Here's how the part is built. I have some questions about the finished solid (model axes, mm). A direction names the side the tool comes from. Coordinates: 2 decimals unless noted, no trailing zeros. Loops run counter-clockwise (first coordinate to the right, second up) from the corner with the lowest first, then second, coordinate; pieces in that order, holes last.
```python
from build123d import *

# Parameters (mm, degrees)
SKETCH_10_W         = 15
SKETCH_10_H         = 8
EXTRUDE_7_DEPTH     = 11
CUT_EXTRUDE_4_DEPTH = 11
SKETCH_12_W         = 15
SKETCH_12_H         = 6
EXTRUDE_8_DEPTH     = 6
SKETCH_14_W         = 15
SKETCH_14_H         = 5
EXTRUDE_9_DEPTH     = 4
EXTRUDE_10_DEPTH    = 15
EXTRUDE_11_DEPTH    = 5
SKETCH_19_R         = 1.1
CUT_EXTRUDE_5_DEPTH = 5
EXTRUDE_START       = 0.5
SKETCH_20_R         = 1.5
SKETCH_20_R_2       = 1.1
EXTRUDE_12_DEPTH    = 0.5
SKETCH_21_R         = 1.5
SKETCH_21_R_2       = 1.1
EXTRUDE_13_DEPTH    = 0.5
FILLET_4_R          = 0.5
CHAMFER_1_SIZE      = 4.493554602
CHAMFER_1_SIZE_2    = 2.7
FILLET_7_R          = 2
SKETCH_22_W         = 15
SKETCH_22_H         = 2
EXTRUDE_14_DEPTH    = 6
FILLET_8_R          = 2
FILLET_9_R          = 2


# Some blends are built 0.0001 mm under size
with BuildPart() as part:
    # 草图10 → 凸台-拉伸7 (new body)
    with BuildSketch(Plane.XY):
        with Locations((0, 24.68211788)):
            Rectangle(SKETCH_10_W, SKETCH_10_H)
    extrude(amount=EXTRUDE_7_DEPTH)

    # 草图11 → 切除-拉伸4 (cut)
    with BuildSketch(Plane(origin=(0, 28.68211788, 0), x_dir=(1, 0, 0), z_dir=(0, 1, 0))):
        with BuildLine():
            Line((-3.45, -5), (-3.45, -7))
            ThreePointArc((-3.45, -7), (-5, -8.55), (-6.55, -7))
            Line((-6.55, -7), (-6.55, -5))
            ThreePointArc((-6.55, -5), (-5, -3.45), (-3.45, -5))
        make_face()
        with BuildLine():
            Line((3.45, -5), (3.45, -7))
            ThreePointArc((3.45, -7), (5, -8.55), (6.55, -7))
            Line((6.55, -7), (6.55, -5))
            ThreePointArc((6.55, -5), (5, -3.45), (3.45, -5))
        make_face()
    extrude(amount=-CUT_EXTRUDE_4_DEPTH, mode=Mode.SUBTRACT)

    # 草图12 → 凸台-拉伸8 (add)
    with BuildSketch(Plane.XY.offset(11)):
        with Locations((0, 25.68211788)):
            Rectangle(SKETCH_12_W, SKETCH_12_H)
    extrude(amount=EXTRUDE_8_DEPTH)

    # 草图14 → 凸台-拉伸9 (add)
    with BuildSketch(Plane.XY.offset(17)):
        with Locations((0, 23.5)):
            Rectangle(SKETCH_14_W, SKETCH_14_H)
    extrude(amount=EXTRUDE_9_DEPTH)

    # 草图17 → 凸台-拉伸10 (add)
    with BuildSketch(Plane.ZY.offset(7.5)):
        Polygon((21, 26), (24.535533906, 29.535533906), (28.071067812, 26), (23.071067812, 21), (21, 21), align=None)
    extrude(amount=-EXTRUDE_10_DEPTH)

    # 草图18 → 凸台-拉伸11 (add)
    with BuildSketch(Plane(origin=(0, -1.035533906, 1.035533906), x_dir=(1, 0, 0), z_dir=(0, -0.7071067811865507, 0.7071067811865445))):
        with BuildLine():
            Line((7.5, 38.234018716), (-7.5, 38.234018716))
            ThreePointArc((-7.5, 38.234018716), (0, 45.734018716), (7.5, 38.234018716))
        make_face()
    extrude(amount=-EXTRUDE_11_DEPTH)

    # 草图19 → 切除-拉伸5 (cut)
    with BuildSketch(Plane(origin=(0, -1.035533906, 1.035533906), x_dir=(1, 0, 0), z_dir=(0, -0.7071067811865507, 0.7071067811865445))):
        with Locations(Location((0, 38.234018716, 0), (0, 0, 270))):
            Circle(SKETCH_19_R)
    extrude(amount=-CUT_EXTRUDE_5_DEPTH, mode=Mode.SUBTRACT)

    # 草图20 → 凸台-拉伸12 (add)
    with BuildSketch(Plane(origin=(0, -1.035533906, 1.035533906), x_dir=(1, 0, 0), z_dir=(0, -0.7071067811865507, 0.7071067811865445)).offset(EXTRUDE_START)):
        with Locations(Location((0, 38.234018716, 0), (0, 0, 270))):
            Circle(SKETCH_20_R)
        with Locations(Location((0, 38.234018716, 0), (0, 0, 270))):
            Circle(SKETCH_20_R_2, mode=Mode.SUBTRACT)
    extrude(amount=-EXTRUDE_12_DEPTH)

    # 草图21 → 凸台-拉伸13 (add)
    with BuildSketch(Plane(origin=(0, 2.5, -2.5), x_dir=(1, 0, 0), z_dir=(0, 0.7071067811865513, -0.7071067811865437))):
        with Locations(Location((0, -38.234018716, 0), (0, 0, 90))):
            Circle(SKETCH_21_R)
        with Locations(Location((0, -38.234018716, 0), (0, 0, 90))):
            Circle(SKETCH_21_R_2, mode=Mode.SUBTRACT)
    extrude(amount=EXTRUDE_13_DEPTH)

    # 圆角4
    fillet_4_edges = [part.edges().sort_by_distance(p)[0] for p in [
        (0, 27.060660172, 29.131727984),
        (0, 30.596194078, 25.596194078),
    ]]
    fillet(fillet_4_edges, radius=FILLET_4_R - 0.0001)  # a hair under: the kernel refuses the full size

    # 倒角1
    # the kernel refuses this chamfer: 4.493554602, 2.7 mm, written as the material it adds along each edge
    with BuildSketch(Plane(origin=(-7.5, 26, 17), x_dir=(0, -0.01991463058083334, 0.9998016840798123), z_dir=(1, 0, 0))) as chamfer_1_piece_1_section:
        Polygon((CHAMFER_1_SIZE * 0.999801684157, -CHAMFER_1_SIZE * 0.0199146305824), (-CHAMFER_1_SIZE_2 * 0.0199146305808, -CHAMFER_1_SIZE_2 * 0.99980168408), (0, 0), align=None)
    chamfer_1_piece_1 = extrude(amount=15, mode=Mode.PRIVATE)
    chamfer_1_piece_1 = split(chamfer_1_piece_1, bisect_by=Plane(origin=(0, 28.68211788, 18.477199106), z_dir=(0, -1, 0)), keep=Keep.TOP, mode=Mode.PRIVATE)
    add(chamfer_1_piece_1)

    # 圆角7
    fillet_7_edges = [part.edges().sort_by_distance(p)[0] for p in [
        (0, 26.18524881, 21.18524881),
        (0, 28.68211788, 17.029760846),
    ]]
    fillet(fillet_7_edges, radius=FILLET_7_R)

    # 草图22 → 凸台-拉伸14 (add)
    with BuildSketch(Plane.XY.offset(11)):
        with Locations((0, 21.68211788)):
            Rectangle(SKETCH_22_W, SKETCH_22_H)
    extrude(amount=EXTRUDE_14_DEPTH)

    # 圆角8
    # the kernel refuses this fillet: 2 mm, written as the material it adds along each edge
    with BuildSketch(Plane(origin=(7.5, 21, 17), x_dir=(0, -1.0, 7.298057631676466e-12), z_dir=(-1, 0, 0))) as fillet_8_piece_1:
        with BuildLine():
            CenterArc((2, 1.08188698), FILLET_8_R, 180, 32.747889427)
            Line((0, 1.08188698), (-0.04, 1.08188698))
            Line((-0.04, 1.08188698), (-0.04, 0))
            Line((-0.04, 0), (0, -0.04))
            ThreePointArc((0, -0.04), (0.15894106, -0.04), (0.284239762, -0.02163774))
            Line((0.284239762, -0.02163774), (0.31788212, 0))
        make_face()
    extrude(amount=15)

    # 圆角9
    fillet_9_edges = [part.edges().sort_by_distance(p)[0] for p in [
        (0, 28.68211788, 0),
    ]]
    fillet(fillet_9_edges, radius=FILLET_9_R)


solid = part.part
```
1. On a 3-axis mill with a long thin cutter (end or side, diameter ignored), from which of +Z, -Z, +X, -X, +Y, -Y can I reach the whole of each face in a straight line? I mean faces 1 (the flat face through (0, 28.682, 9)), 2 (the cylindrical face through (-5.03, 24.74, 3.45)), 3 (the flat face through (1.77, 25.08, 27.15)), 4 (the cylindrical face through (0.105, 28.607, 17.017)). Say none if no direction works.
2. For pin 1 (4 mm diameter, centred on x = -2.5, z = 7.5, fed in from +Y); pin 2 (1.5 mm diameter, centred on x = -2, z = 20.5, fed in from -Y), each with a flat end and sliding along its axis, tell me the tip position at first contact or that it passes through.
3. I want a section at D-D (y = 27.75). Give the number of separate pieces and of enclosed holes in the cut face, then the cut area to 3 significant figures.
4. I want a section at A-A (x = 5). Please give me the cut outline in (y, z), then the cut area to 3 significant figures.
5. I need wall thicknesses on line 1 along Z through (x, y) = (-1.5, 25.25); line 2 along X through (y, z) = (27.25, 4.5); line 3 along Y through (x, z) = (3.5, 9.5). Which ranges of each line are inside material? Lowest first, please.
6. I want a section at B-B (y = 23). Please give me the cut outline in (x, z).
7. I want a section at C-C (z = 15.5). Please give me the cut outline in (x, y).
8. We'd pull the mould along Z, two halves only. Please class faces 5 (the cylindrical face through (-4.97, 24.74, 8.55)), 6 (the flat face through (0, 21, 21)), 7 (the cylindrical face through (0.11, 28.08, 0.57)), 8 (the cylindrical face through (0.105, 20.921, 17.526)): +Z half, -Z half, draft (parallel to the pull), parting line (faces both ways), or undercut.
Response values:
1. face 1: -Z, +X, -X, +Y
1. face 2: +Y, -Y
1. face 3: +Z, -Y
1. face 4: +X, -X, +Y
2. pin 1: stops at y = 28.68
2. pin 2: stops at y = 21
3. separate pieces: 2
3. enclosed holes: 3
3. area: 346 mm2
4. outline: (20.68, 0) - (26.68, 0) arc R2 ccw to (28.68, 2) - (28.68, 3.45) - (20.68, 3.45) - close; (20.68, 8.55) - (28.68, 8.55) - (28.68, 16.48) arc R2 ccw to (28.4, 17.51) - (26.99, 19.85) arc R2 cw to (27.29, 22.29) - (33.49, 28.49) - (29.95, 32.02) - (21, 23.07) - (21, 18.08) arc R2 cw to (20.68, 17) - close
4. area: 184 mm2
5. line 1: z = 0 to 27.37
5. line 2: x = -7.5 to -6.47, -3.53 to 3.53, 6.47 to 7.5
5. line 3: y = 20.68 to 28.68
6. outline: (-7.5, 0) - (7.5, 0) - (7.5, 25.07) - (-7.5, 25.07) - close; hole (-6.55, 5) arc R1.55 ccw to (-3.45, 5) - (-3.45, 7) arc R1.55 ccw to (-6.55, 7) - close; hole (3.45, 5) arc R1.55 ccw to (6.55, 5) - (6.55, 7) arc R1.55 ccw to (3.45, 7) - close
7. outline: (-7.5, 20.68) - (7.5, 20.68) - (7.5, 28.68) - (-7.5, 28.68) - close
8. face 5: undercut
8. face 6: draft
8. face 7: -Z half
8. face 8: +Z half
